Source: CAD feature listing. Evaluate the final solid. Frame: model axes, mm. Face numbers are marked on the shaded views. Give positions to 0.01 mm unless a question says otherwise; leave off trailing zeros. Order: outer loops, then holes, each group sorted by start corner. A loop starts at its lowest first (then second) coordinate and runs counter-clockwise, first axis right, second up.
Autodesk Fusion 360 part; units mm, degrees
sketch "3D-printed conduit outline" plane through (0, 0, 0) normal (0, 1, 0) x (1, 0, 0)
  line L0 (0, 0) -> (16, 0)
  line L1 (16, 0) -> (16, -14)
  line L2 (16, -14) -> (0, -14)
  line L3 (0, -14) -> (0, 0)
  line L4 (2, -14) -> (14, -14)
  line L5 (14, -14) -> (14, -2)
  line L6 (14, -2) -> (2, -2)
  line L7 (2, -2) -> (2, -14)
  dimension "d8" = 14
  dimension "d9" = 16
  dimension "d10" = 2
  dimension "d11" = 2
  dimension "d12" = 2
extrude "Extrude1" add sketch "3D-printed conduit outline" along normal blind 94 contours L0 L1 L2 L3 L5 L6 L7
sketch "Magnet holders" plane through (0, 0, 14) normal (0, 0, 1) x (-1, 0, 0)
  line L0 (0, 0) -> (-2, 0)
  line L1 (-2, 0) -> (-2, -94)
  line L2 (-2, -94) -> (0, -94)
  line L3 (0, -94) -> (0, 0)
  line L4 (-14, 0) -> (-16, 0)
  line L5 (-16, 0) -> (-16, -94)
  line L6 (-16, -94) -> (-14, -94)
  line L7 (-14, -94) -> (-14, 0)
  circle A0 centre (-2.5, -2.5) radius 2.5
  circle A1 centre (-2.5, -2.5) radius 1.75
  line L8 (-14, 0) -> (-2, 0)
  line L9 (0, 0) -> (-2.5, 0)
  line L10 (-2.5, 0) -> (-2.5, -5)
  line L11 (-2.5, -5) -> (0, -5)
  line L12 (0, -5) -> (0, 0)
  circle A2 centre (-13.5, -2.5) radius 2.5
  circle A3 centre (-13.5, -2.5) radius 1.75
  line L13 (-16, 0) -> (-13.5, 0)
  line L14 (-13.5, 0) -> (-13.5, -5)
  line L15 (-13.5, -5) -> (-16, -5)
  line L16 (-16, -5) -> (-16, 0)
  circle A4 centre (-2.5, -91.5) radius 1.75
  circle A5 centre (-2.5, -91.5) radius 2.5
  line L17 (-2.5, -89) -> (-2.5, -94)
  line L18 (-2.5, -94) -> (0, -94)
  line L19 (0, -94) -> (0, -89)
  line L20 (0, -89) -> (-2.5, -89)
  circle A6 centre (-13.5, -75.5) radius 2.5
  circle A7 centre (-13.5, -75.5) radius 1.75
  line L21 (-13.5, -73) -> (-13.5, -78)
  line L22 (-13.5, -78) -> (-16, -78)
  line L23 (-16, -78) -> (-16, -73)
  line L24 (-16, -73) -> (-13.5, -73)
  dimension "d15" = 5
  dimension "d16" = 3.5
  dimension "d17" = 5
  dimension "d18" = 3.5
  dimension "d21" = 0
  dimension "d22" = -89
  dimension "d42" = 0
  dimension "d43" = -73
sketch "End wall" plane through (0, 94, 0) normal (0, 1, 0) x (-1, 0, 0)
  line L0 (-2, 2) -> (-14, 2)
  line L1 (-14, 2) -> (-14, 14)
  line L2 (-14, 14) -> (-16, 14)
  line L3 (-16, 14) -> (-16, 0)
  line L4 (-16, 0) -> (0, 0)
  line L5 (0, 0) -> (0, 14)
  line L6 (0, 14) -> (-2, 14)
  line L7 (-2, 14) -> (-2, 2)
  line L8 (-16, 0) -> (0, 0)
  line L9 (0, 0) -> (0, 14)
  line L10 (0, 14) -> (-16, 14)
  line L11 (-16, 14) -> (-16, 0)
extrude "Extrude8" add sketch "End wall" against normal blind 2
extrude "Extrude2" add sketch "Magnet holders" against normal blind 3 contours A2 A3 L14 | L7 A2 A3 L14 | L7 L8 A2 L13 | L1 A0 L8 L9 | L1 A0 A1 L10 | A0 A1 L10 | L1 A0 A1 L10 | L1 A0 L11 | L1 A1 L10 | A1 L10 | L7 A3 L14 | A3 L14 | L1 A5 L20 | L7 A2 L15 | L7 A2 A3 L14 | L1 A4 A5 L17 | L1 A4 A5 L17 | L1 A5 L18 | A4 A5 L17 | L1 A4 L17 | A4 L17 | L7 A6 L24 | L7 A6 A7 L21 | A6 A7 L21 | L7 A7 L21 | A7 L21 | L7 A6 L22 | L7 A6 A7 L21
extrude "Extrude4" cut sketch "Magnet holders" against normal blind 1 contours L1 A1 | L1 A1 L10 | A1 L10 | L7 A3 L14 | A3 L14 | L7 A3 | L1 A4 | L1 A4 L17 | A4 L17 | L7 A7 L21 | L7 A7 | A7 L21
chamfer "Chamfer2" distance 2.9999 angle 45 4 edges at (2, 2.5, 11) (2, 90.5, 11) (14, 2.5, 11) (14, 75.5, 11)
sketch "LED outlets" plane through (0, 0, 0) normal (-1, 0, 0) x (0, -1, 0)
  line L0 (0, 0) -> (0, 14)
  line L1 (0, 14) -> (-94, 14)
  line L2 (-94, 14) -> (-94, 0)
  line L3 (-94, 0) -> (0, 0)
  line L4 (-49, 14) -> (-39, 14)
  line L5 (-39, 14) -> (-39, 2)
  line L6 (-39, 2) -> (-49, 2)
  line L7 (-49, 2) -> (-49, 14)
  line L8 (-84, 14) -> (-74, 14)
  line L9 (-74, 14) -> (-74, 2)
  line L10 (-74, 2) -> (-84, 2)
  line L11 (-84, 2) -> (-84, 14)
  dimension "d31" = 10
  dimension "d32" = 10
  dimension "d33" = 25
  dimension "d34" = 2
  dimension "d35" = 39
extrude "Extrude5" cut sketch "LED outlets" against normal blind 2 contours L1 L4 L5 L6 L7 | L1 L8 L9 L10 L11
sketch "Arcade butons outlet" plane through (16, 0, 0) normal (1, 0, 0) x (0, 1, 0)
  line L0 (94, 14) -> (0, 14)
  line L1 (0, 14) -> (0, 0)
  line L2 (0, 0) -> (94, 0)
  line L3 (94, 0) -> (94, 14)
  line L4 (80, 14) -> (92, 14)
  line L5 (92, 14) -> (92, 2)
  line L6 (92, 2) -> (80, 2)
  line L7 (80, 2) -> (80, 14)
  dimension "d48" = 2
  dimension "d49" = 2
  dimension "d50" = 12
extrude "Extrude9" cut sketch "Arcade butons outlet" against normal blind 2 contours L0 L4 L5 L6 L7
sketch "Colour sensor outlet" plane through (16, 0, 0) normal (1, 0, 0) x (0, 1, 0)
  line L0 (80, 2) -> (80, 14)
  line L1 (80, 14) -> (0, 14)
  line L2 (0, 14) -> (0, 0)
  line L3 (0, 0) -> (94, 0)
  line L4 (94, 0) -> (94, 14)
  line L5 (94, 14) -> (92, 14)
  line L6 (92, 14) -> (92, 2)
  line L7 (92, 2) -> (80, 2)
  line L8 (28.705, 14) -> (53.917, 14)
  line L9 (53.917, 14) -> (53.917, 2)
  line L10 (53.917, 2) -> (28.705, 2)
  line L11 (28.705, 2) -> (28.705, 14)
  dimension "d54" = 2
  dimension "d55" = 25.212
  dimension "d58" = 28.705
extrude "Extrude10" cut sketch "Colour sensor outlet" against normal blind 2 contours L1 L8 L9 L10 L11
chamfer "Chamfer4" distance 1 angle 45 13 edges at (2, 19.5, 2) (1, 39, 2) (1, 49, 2) (2, 61.5, 2) (1, 74, 2) (1, 84, 2) (2, 88, 2) (9, 92, 2) (15, 80, 2) (14, 66.9585, 2) (15, 53.917, 2) (15, 28.705, 2) (14, 14.3525, 2)
equation "conduit_length = 94 mm"
equation "conduit_width = 16 mm"
equation "conduit_height = 16 mm"
equation "conduit_wall_thickness = 2 mm"
equation "magnet_diameter = 3 mm"
equation "magnet_height = 1 mm"
equation "d8 = conduit_height - conduit_wall_thickness"
equation "d9 = conduit_width"
equation "d10 = conduit_wall_thickness"
equation "d11 = conduit_wall_thickness"
equation "d12 = conduit_wall_thickness"
equation "d13 = conduit_length"
equation "d15 = magnet_diameter + 2 mm"
equation "d16 = magnet_diameter + 0.5 mm"
equation "d17 = magnet_diameter + 2 mm"
equation "d18 = magnet_diameter + 0.5 mm"
equation "d22 = -conduit_length + ( magnet_diameter + 2 mm )"
equation "d23 = -( magnet_height + 2 mm )"
equation "d34 = conduit_wall_thickness"
equation "d43 = -conduit_length + ( magnet_diameter + 2 mm ) + ( conduit_width )"
equation "d48 = conduit_wall_thickness"
equation "d49 = conduit_wall_thickness"
equation "d50 = conduit_width - 2 * conduit_wall_thickness"
equation "d54 = conduit_wall_thickness"
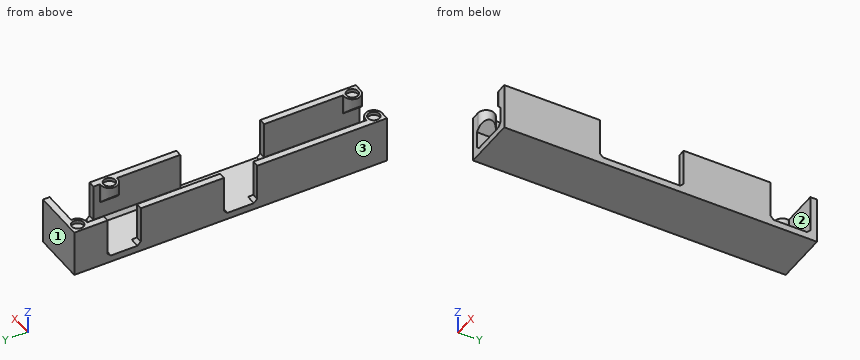
1) Section query D-D, the plane z = 10. Count the separate pieces of the cut face and the enclosed holes in it, and give its area (3 significant figures).
Report:
separate pieces: 5
enclosed holes: 0
area: 320 mm2
2) Section query C-C, the plane y = 87. Return the cut outline in (x, z), and give its area (3 significant figures).
Report:
outline: (0, 0) - (16, 0) - (16, 2) - (3, 2) - (2, 3) - (2, 14) - (0, 14) - close
area: 56.5 mm2
3) Material intervals for L1, parallel to Y at x = 2.5, z = 13.4; L2, parallel to Y at x = 1.75, z = 7; L3, parallel to X at y = 2.5, z = 13.45, sorted ascending.
Report:
L1: y = 0 to 0.75, 4.25 to 5, 89 to 89.75, 93.25 to 94
L2: y = 0 to 39, 49 to 74, 84 to 94
L3: x = 0 to 0.75, 4.25 to 5, 11 to 11.75, 15.25 to 16
4) Pin query (flat end, axial travel): pin 1 (1.8 mm diameter, centred on x = 2.5, y = 2.5, fed in from +Z); pin 2 (3 mm diameter, centred on x = 13, y = 75, fed in from +Z); pin 3 (5 mm diameter, centred on x = 10, y = 54, fed in from +Z); pin 4 (1 mm diameter, centred on y = 36.5, z = 6.5, fed in from +X). Return the tip coordinate at first contact, or that it passes through.
Report:
pin 1: stops at z = 13
pin 2: stops at z = 14
pin 3: stops at z = 2
pin 4: stops at x = 2
5) Section query B-B, the plane x = 9.5. Return the cut outline in (y, z), and give its area (4 significant figures).
Report:
outline: (0, 0) - (94, 0) - (94, 14) - (92, 14) - (92, 3) - (91, 2) - (0, 2) - close
area: 212.5 mm2
6) Section query A-A, the plane y = 71. Return the cut outline in (x, z).
Report:
outline: (0, 0) - (16, 0) - (16, 14) - (14, 14) - (14, 3) - (13, 2) - (3, 2) - (2, 3) - (2, 14) - (0, 14) - close
7) Draft query along Y for the marked faces 1, 2 and 3. Return one class per face: +Y half, -Y half, draft (parallel to the pull), parting line (faces both ways), or undercut.
Report:
face 1: +Y half
face 2: undercut
face 3: draft
